Here's the drawing with two shaded views (mm, measured from the low corner). I have some questions. Coordinates: 2 decimals unless noted, no trailing zeros. Loops run counter-clockwise (first coordinate to the right, second up) from the corner with the lowest first, then second, coordinate; pieces in that order, holes last. Notation, with made-up numbers: (-11, -26.5) -> (11, -26.5) arc R32 ccw to (11, 9.5) -> close; hole circle Ø3 at (37, -5.75). An arc over 180 degrees is marked (long way). Answer as a JSON object with one key per item and string values. Group by question number.
1) I need wall thicknesses on probe 1 along Z at (x, y) = (27, 1.7); probe 2 along Z at (x, y) = (31, 0.6); probe 3 along Y at (x, z) = (27, 14). Which ranges of each line are inside material? Lowest first, please. Write a range as [from, to].
2) I want a section at C-C (y = 0.3). Write out the boundary of the cut face in (x, z), then the cut area to 3 significant figures.
3) I want a section at A-A (z = 10.5). Write out the boundary of the cut face in (x, y).
4) I'm going to push flat-ended pins straight in: pin 1 (1 mm diameter, centred on x = 28.5, y = 0.5, fed in from +Z); pin 2 (0.8 mm diameter, centred on x = 27, y = 0.5, fed in from -Z); pin 3 (6 mm diameter, centred on x = 22.5, z = 16, fed in from +Y). Where does each tip first touch, or does it pass through?
5) I want a section at B-B (x = 31). Write out the boundary of the cut face in (y, z), then the cut area to 3 significant figures.
6) I want a section at D-D (z = 22). Write out the boundary of the cut face in (x, y).
7) If we mould it in two halves opening along X, with no side actions, what happens to the marked faces 1 and 2? For each: +X half, -X half, draft (parallel to the pull), parting line (faces both ways), or undercut.
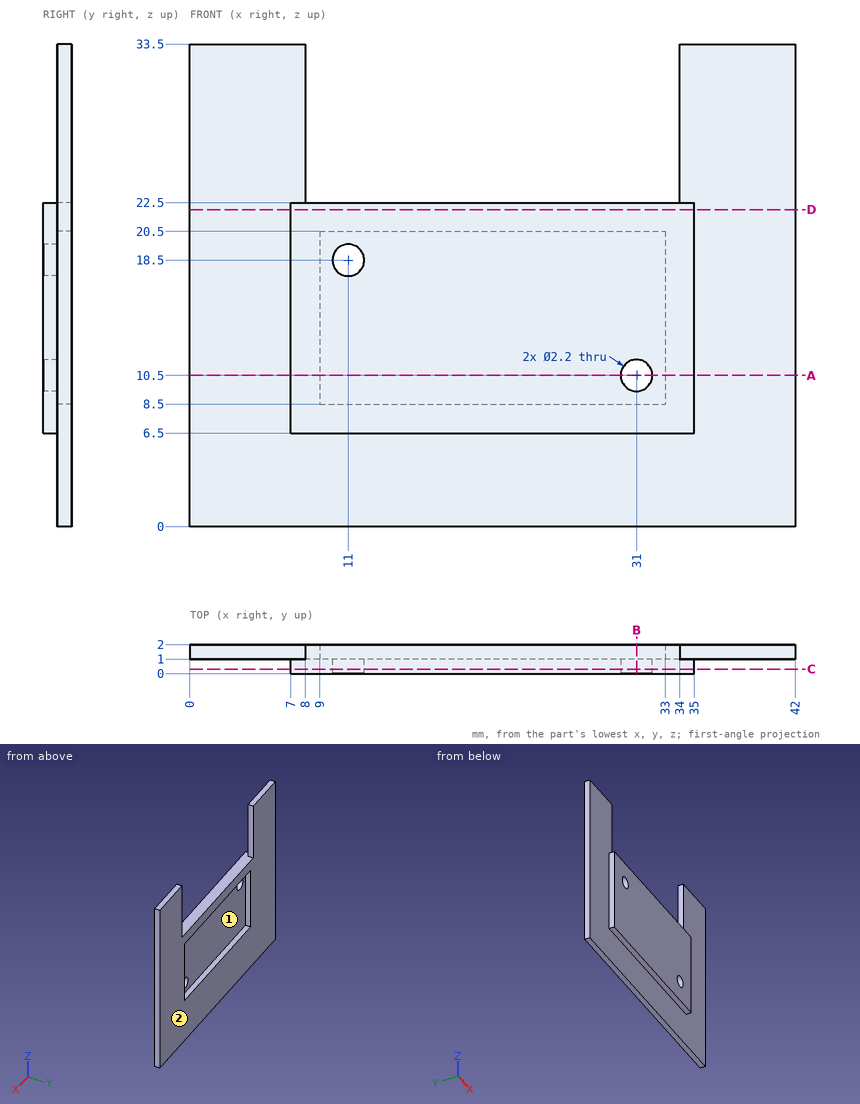
Determined:
{
 "1": {"probe 1": "[0, 8.5], [20.5, 22.5]", "probe 2": "[6.5, 9.4], [11.6, 22.5]", "probe 3": "[0, 1]"},
 "2": {"outline": "(7, 6.5) -> (35, 6.5) -> (35, 22.5) -> (7, 22.5) -> close; hole circle Ø2.2 at (11, 18.5); hole circle Ø2.2 at (31, 10.5)", "area": "440 mm^2"},
 "3": {"outline": "(0, 1) -> (7, 1) -> (7, 0) -> (29.9, 0) -> (29.9, 1) -> (9, 1) -> (9, 2) -> (0, 2) -> close; (32.1, 0) -> (35, 0) -> (35, 1) -> (42, 1) -> (42, 2) -> (33, 2) -> (33, 1) -> (32.1, 1) -> close"},
 "4": {"pin 1": "z = 22.5", "pin 2": "z = 6.5", "pin 3": "y = 1"},
 "5": {"outline": "(0, 6.5) -> (1, 6.5) -> (1, 0) -> (2, 0) -> (2, 8.5) -> (1, 8.5) -> (1, 9.4) -> (0, 9.4) -> close; (0, 11.6) -> (1, 11.6) -> (1, 20.5) -> (2, 20.5) -> (2, 22.5) -> (0, 22.5) -> close", "area": "24.3 mm^2"},
 "6": {"outline": "(0, 1) -> (7, 1) -> (7, 0) -> (35, 0) -> (35, 1) -> (42, 1) -> (42, 2) -> (0, 2) -> close"},
 "7": {"face 1": "undercut", "face 2": "draft"}
}
